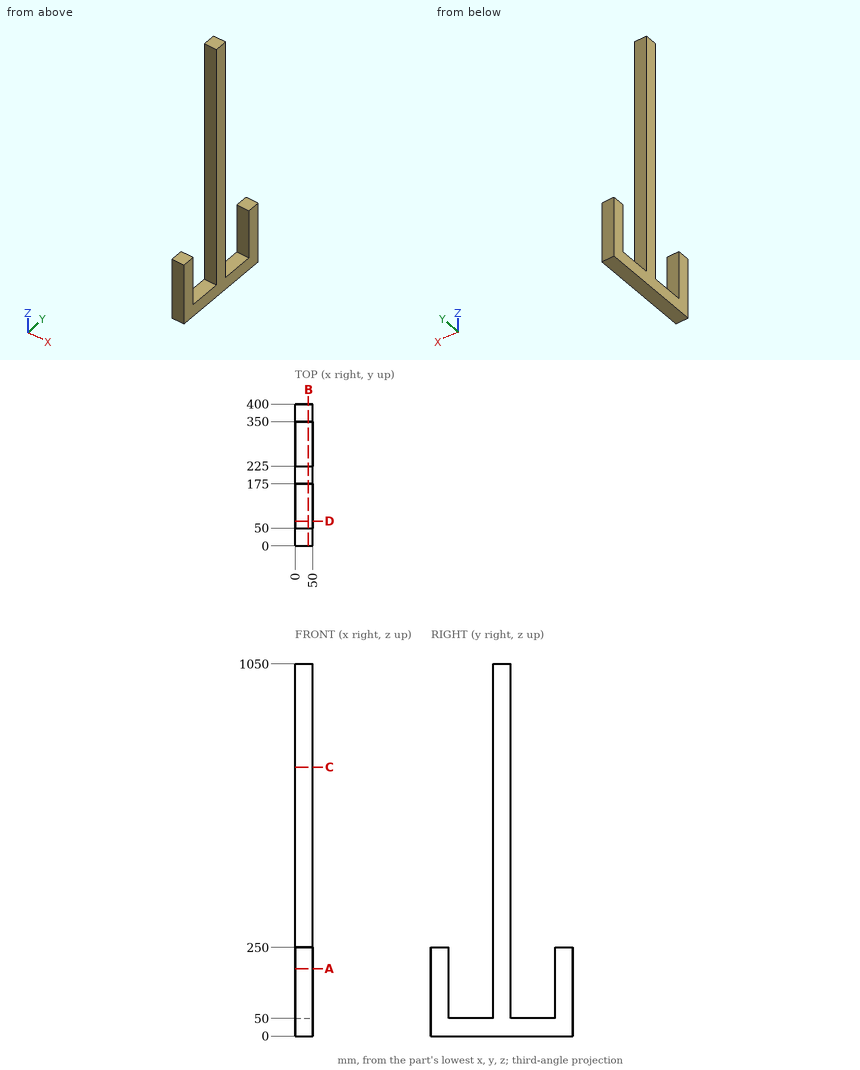
Study the drawing (mm; zero at the part's minimum x, y, z) and answer. Round coordinates to 2 decimals unless told otherwise and drop trailing zeros. Write each loop counter-clockwise with the first axis right and the second up, starting at its lowest first coordinate (ties: lowest second). Pieces come first, ordered by that corner, then holes. Notation, with made-up numbers: (-29.75, -39.5) -> (26.25, -39.5) arc R26 cw to (26.25, -5.5) -> close; hole circle Ø6 at (-31, 8). An arc over 180 degrees is marked (long way). Write each question's results on one line, items separated by ' | '.
Item 1: A cutting plane is placed at B-B, the plane x = 37. Determine the outline of the cut face in (y, z), plus the area to 3 significant figures.
Result set:
outline: (0, 0) -> (400, 0) -> (400, 250) -> (350, 250) -> (350, 50) -> (225, 50) -> (225, 1050) -> (175, 1050) -> (175, 50) -> (50, 50) -> (50, 250) -> (0, 250) -> close | area: 90,000 mm^2
Item 2: Find the intervals of material crossed by line 1 along Y through (x, z) = (47.5, 239); line 2 along Y through (x, z) = (18, 278); line 3 along Z through (x, y) = (22.5, 293), in increasing order. Write a range as [from, to].
Result set:
line 1: [0, 50], [175, 225], [350, 400] | line 2: [175, 225] | line 3: [0, 50]
Item 3: A cutting plane is placed at A-A, the plane z = 190. Determine the outline of the cut face in (x, y).
Result set:
outline: (0, 0) -> (50, 0) -> (50, 50) -> (0, 50) -> close; (0, 175) -> (50, 175) -> (50, 225) -> (0, 225) -> close; (0, 350) -> (50, 350) -> (50, 400) -> (0, 400) -> close
Item 4: A cutting plane is placed at C-C, the plane z = 758.5. Determine the outline of the cut face in (x, y).
Result set:
outline: (0, 175) -> (50, 175) -> (50, 225) -> (0, 225) -> close
Item 5: Flat-ended cylindrical pins translate along their axes: P1, Ø15, axis at x = 23.5, y = 383.5, coming from the +Z side; P2, Ø15, axis at x = 19, y = 269, coming from the +Z side; P3, Ø3, axis at x = 22, z = 429.5, coming from the +Y side. Find the tip coordinate at first contact, or state that the pin passes through.
Result set:
P1: z = 250 | P2: z = 50 | P3: y = 225
Item 6: A cutting plane is placed at D-D, the plane y = 69.5. Determine the outline of the cut face in (x, z).
Result set:
outline: (0, 0) -> (50, 0) -> (50, 50) -> (0, 50) -> close
